The listing builds one solid part. Answer for the finished solid, in the listing's coordinates (mm). A direction names the side the tool comes from. Round coordinates to 2 decimals unless told otherwise and drop trailing zeros. Write each loop counter-clockwise with the first axis right and the second up, starting at its lowest first coordinate (ties: lowest second). Pieces come first, ordered by that corner, then holes. Notation, with made-up numbers: M 45,74 L 82,74 A36 cw 82,110 Z; hole C -1.75,55 d4. An arc over 180 degrees is marked long. One line per item, written item: value. Start each with the question number.
(1) Section C-C (y = 1.5) is taken. Determine the outline of the cut face in (x, z).
(2) Section B-B (x = 0) is taken. Determine the outline of the cut face in (y, z), plus the area to 3 significant figures.
(3) Given P1, Ø1.5, axis at x = 4.5, y = 2, coming from the +Z side; P2, Ø5, axis at x = 5.5, y = 3, coming from the -Z side; P3, Ø4, axis at x = 0.5, y = 5, coming from the -Z side; P4, Ø5, axis at x = 0, z = 0, coming from the +Y side, each flat-ended and moving along its own axis, determine where each tip first touches the part or whether it passes through.
(4) Section A-A (z = 0) is taken. Determine the outline of the cut face in (x, y), plus the area to 3 significant figures.
(5) For a pull along Y with two mould halves and no side action, classify faces 1 (the flat face through (-7, 8, 0)), 2 (the cylindrical face through (7.81, -0.49, 1.73)), 3 (the flat face through (2, 9, 2)) as released by +Y, released by -Y, zero draft, split by the parting line, or undercut.
(6) Section D-D (z = -2.25) is taken. Determine the outline of the cut face in (x, y), plus the area to 3 significant figures.
(7) For faces 4 (the flat face through (2, -1, -2)), 5 (the flat face through (-7, 0, 0)), determine the directions among +Z, -Z, +X, -X, +Y, -Y from which every point of the face is accessible in a straight line to the end or side of a thin tool.
(8) Consider probe 1 along Y at (x, z) = (-4.5, 4.75); probe 2 along X at (y, z) = (1.75, 0); probe 3 along Z at (x, y) = (-0.25, -0.5). Determine where each line is inside the solid, lowest interval first.
```python
from build123d import *

# Parameters (mm, degrees)
SKETCH2_W          = 6.5
SKETCH2_H          = 8
SKETCH2_W_2        = 8
SKETCH2_H_2        = 1
SKETCH4_R          = 2
CUT_EXTRUDE1_DEPTH = 10


with BuildPart() as part:
    # Sketch2 → Revolve1 (revolve)
    with BuildSketch(Plane.XY, mode=Mode.PRIVATE) as revolve1_sk:
        Polygon((-6.5, 8), (0, 8), (0, 9), (-8, 9), (-8, 8), align=None)
        with Locations((-3.25, 4)):
            Rectangle(SKETCH2_W, SKETCH2_H)
        with Locations((-4, -0.5)):
            Rectangle(SKETCH2_W_2, SKETCH2_H_2)
    revolve(revolve1_sk.sketch.rotate(Axis((0, 0, 0), (0, 1, 0)), 270), axis=Axis((0, 0, 0), (0, 1, 0)))

    # Sketch4 → Cut-Extrude1 (cut)
    with BuildSketch(Plane(origin=(0, 9, 0), x_dir=(1, 0, 0), z_dir=(0, 1, 0))):
        with Locations(Location((0, 0, 0), (0, 0, 270))):
            Circle(SKETCH4_R)
    extrude(amount=-CUT_EXTRUDE1_DEPTH, mode=Mode.SUBTRACT)


solid = part.part
```
Recorded:
1. outline: C 0,0 d13; hole C 0,0 d4
2. outline: M -1,-8 L 0,-8 L 0,-6.5 L 8,-6.5 L 8,-8 L 9,-8 L 9,-2 L -1,-2 Z; M -1,2 L 9,2 L 9,8 L 8,8 L 8,6.5 L 0,6.5 L 0,8 L -1,8 Z
2. area: 96.0 mm2
3. P1: stops at z = 5.31
3. P2: stops at z = -5.77
3. P3: stops at z = -6.5
3. P4: stops at y = 9
4. outline: M -8,-1 L -2,-1 L -2,9 L -8,9 L -8,8 L -6.5,8 L -6.5,0 L -8,0 Z; M 2,-1 L 8,-1 L 8,0 L 6.5,0 L 6.5,8 L 8,8 L 8,9 L 2,9 Z
4. area: 96.0 mm2
5. face 1: undercut
5. face 2: zero draft
5. face 3: released by +Y
6. outline: M -7.68,-1 L 7.68,-1 L 7.68,0 L 6.1,0 L 6.1,8 L 7.68,8 L 7.68,9 L -7.68,9 L -7.68,8 L -6.1,8 L -6.1,0 L -7.68,0 Z
6. area: 128 mm2
7. face 4: +Z, -Z, +X, -X, -Y
7. face 5: none
8. probe 1: y = -1 to 0, 8 to 9
8. probe 2: x = -6.5 to -2, 2 to 6.5
8. probe 3: z = -8 to -1.98, 1.98 to 8
